For this review, take the finished solid that the model builds, in its own axes (mm). Coordinates: 2 decimals unless noted, no trailing zeros. Write each loop counter-clockwise with the first axis right and the second up, starting at its lowest first coordinate (ties: lowest second). Pieces come first, ordered by that corner, then holes. Notation, with made-up numbers: (52, -22.5) -> (76, -22.5) arc R20 ccw to (76, -16.5) -> close; hole circle Ø7 at (57, 41). An arc over 180 degrees is marked (long way). One line per item, written item: value. Start each with the question number.
1) Mouldability with a two-part tool opening along Y and no side actions: class faces 1 (the flat face through (0, 5, 0)), 2 (the cylindrical face through (-11.126, -0.028, 14.51)), 3 (the flat face through (0, -5, 0)), 4 (the conical face through (-18, -2.1, 4)) as released by +Y, released by -Y, zero draft, split by the parting line, or undercut.
2) For probe 1 along Y at (x, z) = (13, 13.5); probe 2 along Z at (x, y) = (7, -1); probe 3 along X at (y, z) = (4.5, -5), list the stretches that pass through material, from the lowest coordinate up. Write a range as from..to.
3) Add section A-A (x = 0). State the section outline as (y, z) points.
4) Add section C-C (y = 0.75). State the section outline as (x, z) points.
5) Add section B-B (z = 0). State the section outline as (x, y) points.
6) For pin 1 Ø6 at (y, z) = (-2, 11.5) entering from +X; pin 2 Ø1.5 at (y, z) = (0.5, -14) entering from -X; pin 3 Ø1 at (x, y) = (10.5, 1.5) entering from -Z, all flat-tipped, find the tip position at first contact; note any pin that passes through.
from build123d import *

# Parameters (mm, degrees)
SKETCH2_R           = 20
BOSS_EXTRUDE1_DEPTH = 5


with BuildPart() as part:
    # Sketch2 → Boss-Extrude1 (new body, symmetric)
    with BuildSketch(Plane(origin=(0, 0, 0), x_dir=(1, 0, 0), z_dir=(0, 1, 0))):
        Circle(SKETCH2_R)
    extrude(amount=BOSS_EXTRUDE1_DEPTH, both=True)

    # Sketch3 → Cut-Revolve1 (revolve, cut)
    with BuildSketch(Plane(origin=(0, 0, 0), x_dir=(0, 0, -1), z_dir=(1, 0, 0))):
        Polygon((20, 3), (18.284475438, 2.009541432), (18.284475438, -2.009541432), (20, -3), align=None)
    revolve(axis=Axis((0, 7.747762259, 0), (0, -1, 0)), mode=Mode.SUBTRACT)


solid = part.part
Numbers:
1. face 1: released by +Y
1. face 2: undercut
1. face 3: released by -Y
1. face 4: undercut
2. probe 1: -5..-2.27, 2.27..5
2. probe 2: -16.89..16.89
2. probe 3: -19.36..19.36
3. outline: (-5, -20) -> (-3, -20) -> (-2.01, -18.28) -> (2.01, -18.28) -> (3, -20) -> (5, -20) -> (5, 20) -> (3, 20) -> (2.01, 18.28) -> (-2.01, 18.28) -> (-3, 20) -> (-5, 20) -> close
4. outline: circle Ø36.57 at (0, 0)
5. outline: (-20, -5) -> (20, -5) -> (20, -3) -> (18.28, -2.01) -> (18.28, 2.01) -> (20, 3) -> (20, 5) -> (-20, 5) -> (-20, 3) -> (-18.28, 2.01) -> (-18.28, -2.01) -> (-20, -3) -> close
6. pin 1: x = 18.02
6. pin 2: x = -12.6
6. pin 3: z = -15.31
